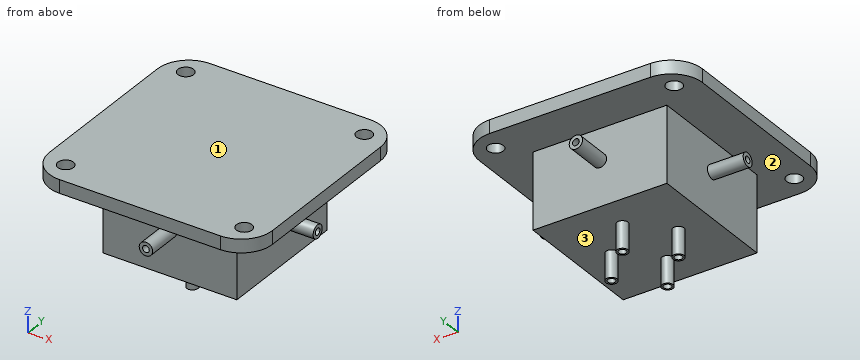
from build123d import *

# Parameters (mm, degrees)
SKETCH_1_R               = 1.75
EXTRUDE_3_DEPTH          = 3
SKETCH_2_W               = 30
SKETCH_2_H               = 30
EXTRUDE_4_DEPTH          = 17
SKETCH_4_R               = 0.75
CUT_EXTRUDE_4_DEPTH      = 9
SKETCH_5_R               = 0.75
CUT_EXTRUDE_5_DEPTH      = 9
SKETCH_17_R              = 0.75
CUT_EXTRUDE_6_DEPTH      = 9
SKETCH_19_R              = 0.75
CUT_EXTRUDE_7_DEPTH      = 9
SKETCH_6_R               = 1.5
SKETCH_6_R_2             = 0.75
EXTRUDE_7_DEPTH          = 8
PATTERN_CIRCULAR_1_COUNT = 4
SKETCH_3_R               = 0.85
CUT_EXTRUDE_8_DEPTH      = 11
SKETCH_21_R              = 1.25
SKETCH_21_R_2            = 0.85
EXTRUDE_8_DEPTH          = 6


with BuildPart() as part:
    # 草图1 → 凸台-拉伸3 (new body)
    with BuildSketch(Plane.XY):
        with BuildLine():
            Line((-18, -25), (18, -25))
            ThreePointArc((18, -25), (22.949747468, -22.949747468), (25, -18))
            Line((25, -18), (25, 18))
            ThreePointArc((25, 18), (22.949747468, 22.949747468), (18, 25))
            Line((18, 25), (-18, 25))
            ThreePointArc((-18, 25), (-22.949747468, 22.949747468), (-25, 18))
            Line((-25, 18), (-25, -18))
            ThreePointArc((-25, -18), (-22.949747468, -22.949747468), (-18, -25))
        make_face()
        with Locations((20, 20)):
            Circle(SKETCH_1_R, mode=Mode.SUBTRACT)
        with Locations((-20, 20)):
            Circle(SKETCH_1_R, mode=Mode.SUBTRACT)
        with Locations((-20, -20)):
            Circle(SKETCH_1_R, mode=Mode.SUBTRACT)
        with Locations((20, -20)):
            Circle(SKETCH_1_R, mode=Mode.SUBTRACT)
    extrude(amount=EXTRUDE_3_DEPTH)

    # 草图2 → 凸台-拉伸4 (add)
    with BuildSketch(Plane.XY):
        Rectangle(SKETCH_2_W, SKETCH_2_H)
    extrude(amount=-EXTRUDE_4_DEPTH)

    # 草图4 → 切除-拉伸4 (cut)
    with BuildSketch(Plane.ZY.offset(15)):
        with Locations((-7, 0)):
            Circle(SKETCH_4_R)
    extrude(amount=-CUT_EXTRUDE_4_DEPTH, mode=Mode.SUBTRACT)

    # 草图5 → 切除-拉伸5 (cut)
    with BuildSketch(Plane(origin=(0, 15, 0), x_dir=(1, 0, 0), z_dir=(0, 1, 0))):
        with Locations((0, 7)):
            Circle(SKETCH_5_R)
    extrude(amount=-CUT_EXTRUDE_5_DEPTH, mode=Mode.SUBTRACT)

    # 草图17 → 切除-拉伸6 (cut)
    with BuildSketch(Plane(origin=(15, 0, 0), x_dir=(0, 0, -1), z_dir=(1, 0, 0))):
        with Locations((7, 0)):
            Circle(SKETCH_17_R)
    extrude(amount=-CUT_EXTRUDE_6_DEPTH, mode=Mode.SUBTRACT)

    # 草图19 → 切除-拉伸7 (cut)
    with BuildSketch(Plane.XZ.offset(15)):
        with Locations((0, -7)):
            Circle(SKETCH_19_R)
    extrude(amount=-CUT_EXTRUDE_7_DEPTH, mode=Mode.SUBTRACT)

    # 草图6 → 凸台-拉伸7 (add)
    with BuildSketch(Plane.ZY.offset(15)):
        with Locations((-7, 0)):
            Circle(SKETCH_6_R)
        with Locations((-7, 0)):
            Circle(SKETCH_6_R_2, mode=Mode.SUBTRACT)
    extrude_7 = extrude(amount=EXTRUDE_7_DEPTH)

    # 阵列(圆周)1: 凸台-拉伸7 ×4 about axis
    pattern_circular_1_axis = Axis((0, 0, 0), (0, 0, 1))
    for i in range(1, PATTERN_CIRCULAR_1_COUNT):
        add(extrude_7.rotate(pattern_circular_1_axis, i * 360 / PATTERN_CIRCULAR_1_COUNT))

    # 草图3 → 切除-拉伸8 (cut)
    with BuildSketch(Plane(origin=(0, 0, -17), x_dir=(-1, 0, 0), z_dir=(0, 0, -1))):
        with Locations((0, -7.5)):
            Circle(SKETCH_3_R)
        with Locations((-7.5, 0)):
            Circle(SKETCH_3_R)
        with Locations((0, 7.5)):
            Circle(SKETCH_3_R)
        with Locations((7.5, 0)):
            Circle(SKETCH_3_R)
    extrude(amount=-CUT_EXTRUDE_8_DEPTH, mode=Mode.SUBTRACT)

    # 草图21 → 凸台-拉伸8 (add)
    with BuildSketch(Plane(origin=(0, 0, -17), x_dir=(-1, 0, 0), z_dir=(0, 0, -1))):
        with Locations((-7.5, 0)):
            Circle(SKETCH_21_R)
        with Locations((-7.5, 0)):
            Circle(SKETCH_21_R_2, mode=Mode.SUBTRACT)
        with Locations((0, -7.5)):
            Circle(SKETCH_21_R)
        with Locations((0, -7.5)):
            Circle(SKETCH_21_R_2, mode=Mode.SUBTRACT)
        with Locations((7.5, 0)):
            Circle(SKETCH_21_R)
        with Locations((7.5, 0)):
            Circle(SKETCH_21_R_2, mode=Mode.SUBTRACT)
        with Locations((0, 7.5)):
            Circle(SKETCH_21_R)
        with Locations((0, 7.5)):
            Circle(SKETCH_21_R_2, mode=Mode.SUBTRACT)
    extrude(amount=EXTRUDE_8_DEPTH)


solid = part.part
CAD build for the part. Positions are in the model's coordinates, mm. Face numbers are marked on the shaded views. A direction names the side the tool comes from. Give positions to 0.01 mm unless a question says otherwise; leave off trailing zeros. Order: outer loops, then holes, each group sorted by start corner. A loop starts at its lowest first (then second) coordinate and runs counter-clockwise, first axis right, second up. Notation, with made-up numbers: (45.5, -17.5) -> (49.5, -17.5) arc R15 ccw to (49.5, -9.5) -> close; hole circle Ø4 at (52, 24.5). An arc over 180 degrees is marked (long way). Return JSON: item names as keys, results as strings.
Q1. Drill centre lines: line 1 (Z direction, x = 0, y = -21); line 2 (Y direction, x = 12, z = -7); line 3 (X direction, y = 18.25, z = -7). Where is each one in solid material? Low to high.
Working result:
{"line 1": "-8.5 to -7.75, -6.25 to -5.5, 0 to 3", "line 2": "-15 to -0.75, 0.75 to 15", "line 3": "-1.5 to -0.75, 0.75 to 1.5"}
Q2. Saw through at D-D (z = 1.25). Write the cut outline in (x, y).
Working result:
{"outline": "(-25, -18) arc R7 ccw to (-18, -25) -> (18, -25) arc R7 ccw to (25, -18) -> (25, 18) arc R7 ccw to (18, 25) -> (-18, 25) arc R7 ccw to (-25, 18) -> close; hole circle Ø3.5 at (-20, -20); hole circle Ø3.5 at (-20, 20); hole circle Ø3.5 at (20, -20); hole circle Ø3.5 at (20, 20)"}
Q3. Which spindle directions (+Z, -Z, +X, -X, +Y, -Y) get a long thin tool onto all of the face, cutting with end or side? Do the marked faces 1, 2 and 3. Say none if no direction does.
Working result:
{"face 1": "+Z, +X, -X, +Y, -Y", "face 2": "none", "face 3": "-Z"}
Q4. Saw through at B-B (x = -20). Write the cut outline in (y, z).
Working result:
{"outline": "(-24.71, 0) -> (-21.75, 0) -> (-21.75, 3) -> (-24.71, 3) -> close; (-18.25, 0) -> (18.25, 0) -> (18.25, 3) -> (-18.25, 3) -> close; circle Ø3 at (0, -7); (21.75, 0) -> (24.71, 0) -> (24.71, 3) -> (21.75, 3) -> close; hole circle Ø1.5 at (0, -7)"}
Q5. Saw through at A-A (z = -18.25). Write the cut outline in (x, y).
Working result:
{"outline": "circle Ø2.5 at (-7.5, 0); circle Ø2.5 at (0, -7.5); circle Ø2.5 at (0, 7.5); circle Ø2.5 at (7.5, 0); hole circle Ø1.7 at (-7.5, 0); hole circle Ø1.7 at (0, -7.5); hole circle Ø1.7 at (0, 7.5); hole circle Ø1.7 at (7.5, 0)"}
Q6. Flat gauge pins, fed straight in: pin 1 (0.9 mm diameter, centred on y = 0, z = -7, fed in from -X); pin 2 (1.4 mm diameter, centred on x = 0, z = -7, fed in from -Y); pin 3 (1.7 mm diameter, centred on y = 0, z = -7, fed in from +X). Where does each tip first touch, or does it go through?
Working result:
{"pin 1": "x = -6", "pin 2": "y = -6", "pin 3": "x = 23"}
